```python
from build123d import *

# Parameters (mm, degrees)
ESBO_O1_W                  = 50
ESBO_O1_H                  = 50
RESSALTO_EXTRUS_O1_DEPTH   = 5
ESBO_O2_R                  = 15.6
CORTE_EXTRUS_O1_DEPTH      = 8
CORTE_EXTRUS_O1_DEPTH_BACK = 14
ESBO_O3_W                  = 50.011024838
ESBO_O3_H                  = 5
RESSALTO_EXTRUS_O2_DEPTH   = 50
FILETE1_R                  = 3
ESBO_O5_R                  = 2
CORTE_EXTRUS_O4_DEPTH      = 14


with BuildPart() as part:
    # Esboço1 → Ressalto-extrusão1 (new body)
    with BuildSketch(Plane.XY):
        with Locations((25, 25)):
            Rectangle(ESBO_O1_W, ESBO_O1_H)
    extrude(amount=RESSALTO_EXTRUS_O1_DEPTH)

    # Esboço2 → Corte-extrusão1 (cut, two sides)
    with BuildSketch(Plane.XY) as corte_extrus_o1_sk:
        with Locations((25, 25)):
            Circle(ESBO_O2_R)
    extrude(amount=CORTE_EXTRUS_O1_DEPTH, mode=Mode.SUBTRACT)
    extrude(corte_extrus_o1_sk.sketch, amount=-CORTE_EXTRUS_O1_DEPTH_BACK, mode=Mode.SUBTRACT)

    # Esboço3 → Ressalto-extrusão2 (add)
    with BuildSketch(Plane.XY):
        with Locations((25.005512419, -2.5)):
            Rectangle(ESBO_O3_W, ESBO_O3_H)
    extrude(amount=RESSALTO_EXTRUS_O2_DEPTH)

    # Filete1
    filete1_edges = [part.edges().sort_by_distance(p)[0] for p in [
        (25, 0, 5),
    ]]
    fillet(filete1_edges, radius=FILETE1_R)

    # Esboço5 → Corte-extrusão4 (cut)
    with BuildSketch(Plane(origin=(0, 0, 0), x_dir=(1, 0, 0), z_dir=(0, 1, 0))):
        with Locations((25.002756209, -29)):
            Circle(ESBO_O5_R)
    extrude(amount=-CORTE_EXTRUS_O4_DEPTH, mode=Mode.SUBTRACT)


solid = part.part
```
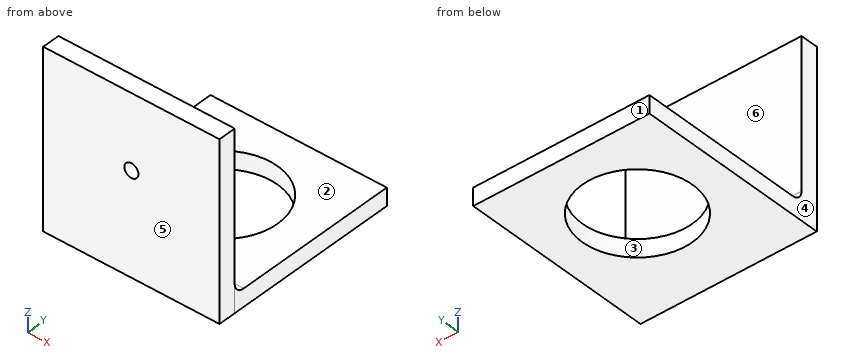
Source: CAD feature listing. Evaluate the final solid. Frame: model axes, mm. Face numbers are marked on the shaded views. A direction names the side the tool comes from. Round coordinates to 2 decimals unless told otherwise and drop trailing zeros. Loops run counter-clockwise (first coordinate to the right, second up) from the corner with the lowest first, then second, coordinate; pieces in that order, holes last.
(1) Section query D-D (x = 31). Output: boundary loops of the cut face in (y, z).
From the geometry:
outline: (-5, 0) - (10.6, 0) - (10.6, 5) - (3, 5) arc R3 cw to (0, 8) - (0, 50) - (-5, 50) - close; (39.4, 0) - (50, 0) - (50, 5) - (39.4, 5) - close
(2) Section query C-C (y = 31). Output: boundary loops of the cut face in (x, z).
From the geometry:
outline: (0, 0) - (10.6, 0) - (10.6, 5) - (0, 5) - close; (39.4, 0) - (50, 0) - (50, 5) - (39.4, 5) - close
(3) Material intervals for probe 1 along X at (y, z) = (-3, 29); probe 2 along Y at (x, z) = (25, 3); probe 3 along Z at (x, y) = (45.5, 46), sorted ascending.
From the geometry:
probe 1: x = 0 to 23, 27 to 50.01
probe 2: y = -5 to 9.4, 40.6 to 50
probe 3: z = 0 to 5
(4) Pull-direction query (Y, two-part tool) for the marked faces 3, 4, 5 and 6; classes: +Y half, -Y half, draft (parallel to the pull), parting line (faces both ways), or undercut.
From the geometry:
face 3: undercut
face 4: draft
face 5: -Y half
face 6: +Y half
(5) Section query A-A (z = 29). Output: boundary loops of the cut face in (x, y).
From the geometry:
outline: (0, -5) - (23, -5) - (23, 0) - (0, 0) - close; (27, -5) - (50.01, -5) - (50.01, 0) - (27, 0) - close
(6) Access query for the marked faces 1 and 2. Directions: +Z, -Z, +X, -X, +Y, -Y. A direction counts if a zero-diameter tool reaches every point of the face in a straight line with its end or side. Return the directions, or none.
From the geometry:
face 1: +Z, -Z, +X, -X, +Y
face 2: +Z, +X, -X, +Y
(7) Section query B-B (x = 25). Output: boundary loops of the cut face in (y, z), and give its area (3 significant figures).
From the geometry:
outline: (-5, 0) - (9.4, 0) - (9.4, 5) - (3, 5) arc R3 cw to (0, 8) - (0, 27) - (-5, 27) - close; (-5, 31) - (0, 31) - (0, 50) - (-5, 50) - close; (40.6, 0) - (50, 0) - (50, 5) - (40.6, 5) - close
area: 326 mm2
(8) Contact query for flat-ended pins moving along their axis: pin 1 Ø25 at (x, z) = (17, 35.5) entering from +Y; pin 2 Ø23.5 at (x, y) = (35, 35) entering from +Z; pin 3 Ø4 at (y, z) = (27, 3.5) entering from +X. Output: stop coordinate, or through.
From the geometry:
pin 1: stops at y = 0
pin 2: stops at z = 5
pin 3: stops at x = 50
